Could you check a few things on this model? Use its own coordinates, in mm. Face numbers are marked on the shaded views. A direction names the side the tool comes from. Give positions to 0.01 mm unless a question says otherwise; leave off trailing zeros. Order: outer loops, then holes, each group sorted by start corner. A loop starts at its lowest first (then second) coordinate and runs counter-clockwise, first axis right, second up.
(1) Imagine slicing it at B-B, the plane y = -5.5. Write out the boundary of the cut face in (x, z), then the cut area to 3 significant figures.
(2) On a 3-axis mill with a long thin cutter (end or side, diameter ignored), from which of +Z, -Z, +X, -X, +Y, -Y can I reach the whole of each face in a straight line? I mean the marked faces 1, 2 and 3. Say none if no direction works.
(3) If we mould it in two halves opening along Z, with no side actions, what happens to the marked faces 4, 5, 6 and 7? For each: released by +Z, released by -Z, zero draft, split by the parting line, or undercut.
(4) Imagine slicing it at C-C, the plane x = 2.5. Write out the boundary of the cut face in (y, z), then the cut area to 3 significant figures.
(5) Imagine slicing it at A-A, the plane y = 0. Write out the boundary of the cut face in (x, z) (1 decimal).
(6) If I drill on probe 1 along Z at (x, y) = (0.75, -4.5); probe 2 along Z at (x, y) = (-3, 4.5); probe 3 along X at (y, z) = (1.75, -21.75), over which ranges is the centre line in solid material (lowest first)?
(7) Imagine slicing it at D-D, the plane y = 4.5. Write out the boundary of the cut face in (x, z).
(8) Will these pins go through, and if not, where does the flat tip stop? pin 1 (10 mm diameter, centred on y = 6.5, z = -3.5, fed in from -X); pin 2 (8 mm diameter, centred on x = 4.5, z = -11.5, fed in from +Y); pin 3 (5 mm diameter, centred on y = 0.5, z = -22, fed in from -X); pin 4 (1 mm diameter, centred on x = 4.5, z = -2.5, fed in from +Y).
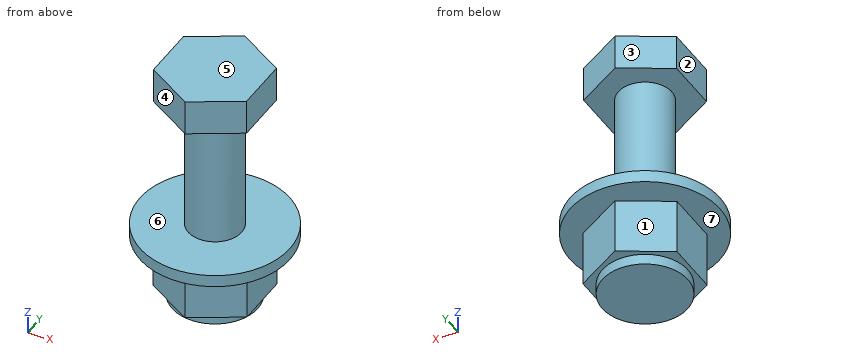
from build123d import *

# Parameters (mm, degrees)
F0_R     = 3.175
F1_DEPTH = 25.4
F3_DEPTH = 4.191
F5_DEPTH = 7.874
F6_R     = 8.89
F7_DEPTH = 1.4478
F8_R     = 5.08
F9_DEPTH = 1.27


with BuildPart() as f1:
    # F0 (on Top) → F1 (new body)
    with BuildSketch(Plane.XY):
        Circle(F0_R)
    extrude(amount=-F1_DEPTH)

    # F2 (on face) → F3 (join)
    with BuildSketch(Plane.XY):
        Polygon((5.5245, 3.189572), (0, 6.379143), (-5.5245, 3.189572), (-5.5245, -3.189572), (0, -6.379143), (5.5245, -3.189572), align=None)
    extrude(amount=F3_DEPTH)

    # F4 (on face) → F5 (join)
    with BuildSketch(Plane(origin=(0, 0, -25.4), x_dir=(1, 0, 0), z_dir=(0, 0, -1))):
        Polygon((5.588, 3.226233), (0, 6.452467), (-5.588, 3.226233), (-5.588, -3.226233), (0, -6.452467), (5.588, -3.226233), align=None)
    extrude(amount=-F5_DEPTH)

    # F6 (on face) → F7 (join)
    with BuildSketch(Plane.XY.offset(-17.526)):
        Circle(F6_R)
    extrude(amount=F7_DEPTH)

    # F8 (on face) → F9 (cut)
    with BuildSketch(Plane(origin=(0, 0, -25.4), x_dir=(1, 0, 0), z_dir=(0, 0, -1))):
        Polygon((5.588, -3.226233), (5.588, 3.226233), (0, 6.452467), (-5.588, 3.226233), (-5.588, -3.226233), (0, -6.452467), align=None)
        Circle(F8_R, mode=Mode.SUBTRACT)
    extrude(amount=-F9_DEPTH, mode=Mode.SUBTRACT)


solid = f1.part
Answer block:
1. outline: (-6.98, -17.53) - (-1.65, -17.53) - (-1.65, -24.13) - (1.65, -24.13) - (1.65, -17.53) - (6.98, -17.53) - (6.98, -16.08) - (-6.98, -16.08) - close; (-1.52, 0) - (1.52, 0) - (1.52, 4.19) - (-1.52, 4.19) - close
1. area: 54.8 mm2
2. face 1: -Z, -X, +Y
2. face 2: +Z, -X, +Y, -Y
2. face 3: +Z, -X, +Y
3. face 4: zero draft
3. face 5: released by +Z
3. face 6: undercut
3. face 7: released by -Z
4. outline: (-8.53, -17.53) - (-5.01, -17.53) - (-5.01, -24.13) - (-4.42, -24.13) - (-4.42, -25.4) - (4.42, -25.4) - (4.42, -24.13) - (5.01, -24.13) - (5.01, -17.53) - (8.53, -17.53) - (8.53, -16.08) - (1.96, -16.08) - (1.96, 0) - (4.94, 0) - (4.94, 4.19) - (-4.94, 4.19) - (-4.94, 0) - (-1.96, 0) - (-1.96, -16.08) - (-8.53, -16.08) - close
4. area: 206 mm2
5. outline: (-8.9, -17.5) - (-5.6, -17.5) - (-5.6, -24.1) - (-5.1, -24.1) - (-5.1, -25.4) - (5.1, -25.4) - (5.1, -24.1) - (5.6, -24.1) - (5.6, -17.5) - (8.9, -17.5) - (8.9, -16.1) - (3.2, -16.1) - (3.2, 0) - (5.5, 0) - (5.5, 4.2) - (-5.5, 4.2) - (-5.5, 0) - (-3.2, 0) - (-3.2, -16.1) - (-8.9, -16.1) - close
6. probe 1: z = -25.4 to -16.08, 0 to 4.19
6. probe 2: z = -24.13 to -16.08, 0 to 4.19
6. probe 3: x = -5.59 to 5.59
7. outline: (-7.67, -17.53) - (-3.38, -17.53) - (-3.38, -24.13) - (-2.36, -24.13) - (-2.36, -25.4) - (2.36, -25.4) - (2.36, -24.13) - (3.38, -24.13) - (3.38, -17.53) - (7.67, -17.53) - (7.67, -16.08) - (-7.67, -16.08) - close; (-3.25, 0) - (3.25, 0) - (3.25, 4.19) - (-3.25, 4.19) - close
8. pin 1: stops at x = -5.52
8. pin 2: stops at y = 3.14
8. pin 3: stops at x = -5.59
8. pin 4: passes through
